Geometry: final body of the model. Coordinates: model frame, mm. Face numbers are marked on the shaded views. A direction names the side the tool comes from. Give positions to 0.01 mm unless a question says otherwise; leave off trailing zeros. Write each loop counter-clockwise with the first axis right and the second up, starting at its lowest first coordinate (ties: lowest second). Pieces come first, ordered by that corner, then holes. Notation, with made-up numbers: (-34.5, -18.5) -> (0.5, -18.5) arc R20 cw to (0.5, 11.5) -> close; hole circle Ø1 at (74, -32.5). An arc over 180 degrees is marked (long way). Answer in a Markdown table with one row per item. Add a question column.
Item 1: Section query A-A on z = 4.75. Output: boundary loops of the cut face in (x, y), plus the area to 3 significant figures.
Item 2: First-contact query: P1, Ø3, axis at x = 2.5, z = 4.5, coming from the -Y side; P2, Ø1, axis at y = -7, z = 2, coming from the -X side; P3, Ø2.5, axis at x = -20, z = 2, coming from the -Y side. Flat tips, straight axial feed; report the tip coordinate or a pass-through.
Item 3: Material intervals for probe 1 along Y at (x, z) = (-33, 3); probe 2 along X at (y, z) = (-2.5, 4.25); probe 3 along X at (y, z) = (-0.75, 2.75), sorted ascending. Write a range as from..to.
Item 4: Section query C-C on x = -7.5. Output: boundary loops of the cut face in (y, z), plus the area to 3 significant figures.
Item 5: Draft query along X for the marked faces 1, 2 and 3. Return one class per face: +X half, -X half, draft (parallel to the pull), parting line (faces both ways), or undercut.
Item 6: Section query B-B on y = -1.5. Output: boundary loops of the cut face in (x, z).
Item 7: Section query D-D on y = -5.5. Output: boundary loops of the cut face in (x, z).
Item 8: Access query for the marked faces 4, 5 and 6. Directions: +Z, -Z, +X, -X, +Y, -Y. A direction counts if a zero-diameter tool reaches every point of the face in a straight line with its end or side. Return the directions, or none.
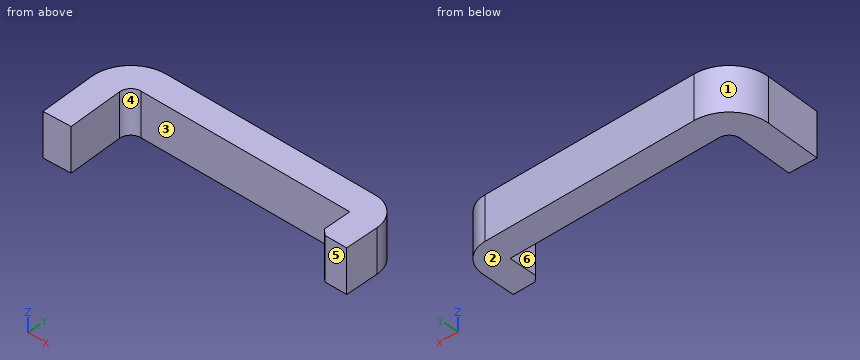
```python
from build123d import *

# Parameters (mm, degrees)
F1_DEPTH = 8
F2_SIZE  = 1
F3_R     = 7
F4_R     = 5


with BuildPart() as f1:
    # F0 (on Top) → F1 (new body)
    with BuildSketch(Plane.XY):
        with BuildLine():
            Line((-44.996954, -12.174497), (-40, -12))
            Line((-40, -12), (-40.34677, -2.069799))
            ThreePointArc((-40.34677, -2.069799), (-39.786668, -0.610683), (-38.347989, 0))
            Line((-38.347989, 0), (0, 0))
            Line((0, 0), (0, -6))
            Line((0, -6), (5, -6))
            Line((5, -6), (5, 5))
            Line((5, 5), (-45.596701, 5))
            Line((-45.596701, 5), (-44.996954, -12.174497))
        make_face()
    extrude(amount=F1_DEPTH)

    # F2
    f2_edges = [f1.edges().sort_by_distance(p)[0] for p in [
        (0, -6, 4),
    ]]
    chamfer(f2_edges, length=F2_SIZE)

    # F3
    f3_edges = [f1.edges().sort_by_distance(p)[0] for p in [
        (-45.596701, 5, 4),
    ]]
    fillet(f3_edges, radius=F3_R)

    # F4
    f4_edges = [f1.edges().sort_by_distance(p)[0] for p in [
        (5, 5, 4),
    ]]
    fillet(f4_edges, radius=F4_R)


solid = f1.part
```
Findings below:
| question | item | result |
|---|---|---|
| 1 | outline | (-45.34, -2.24) -> (-45, -12.17) -> (-40, -12) -> (-40.35, -2.07) arc R2 cw to (-38.35, 0) -> (0, 0) -> (0, -5) -> (1, -6) -> (5, -6) -> (5, 0) arc R5 ccw to (0, 5) -> (-38.35, 5) arc R7 ccw to start |
| 1 | area | 327 mm^2 |
| 2 | P1 | stops at y = -6 |
| 2 | P2 | stops at x = -45.2 |
| 2 | P3 | stops at y = 0 |
| 3 | probe 1 | y = 0..5 |
| 3 | probe 2 | x = -45.33..-40.33, 0..5 |
| 3 | probe 3 | x = -45.24..-39.91, 0..5 |
| 4 | outline | (0, 0) -> (5, 0) -> (5, 8) -> (0, 8) -> close |
| 4 | area | 40.0 mm^2 |
| 5 | face 1 | -X half |
| 5 | face 2 | draft |
| 5 | face 3 | undercut |
| 6 | outline | (-45.33, 0) -> (-40.28, 0) -> (-40.28, 8) -> (-45.33, 8) -> close; (0, 0) -> (5, 0) -> (5, 8) -> (0, 8) -> close |
| 7 | outline | (-45.23, 0) -> (-40.23, 0) -> (-40.23, 8) -> (-45.23, 8) -> close; (0.5, 0) -> (5, 0) -> (5, 8) -> (0.5, 8) -> close |
| 8 | face 4 | +Z, -Z |
| 8 | face 5 | +Z, -Z, +X, -Y |
| 8 | face 6 | +Z, -Z, -Y |
